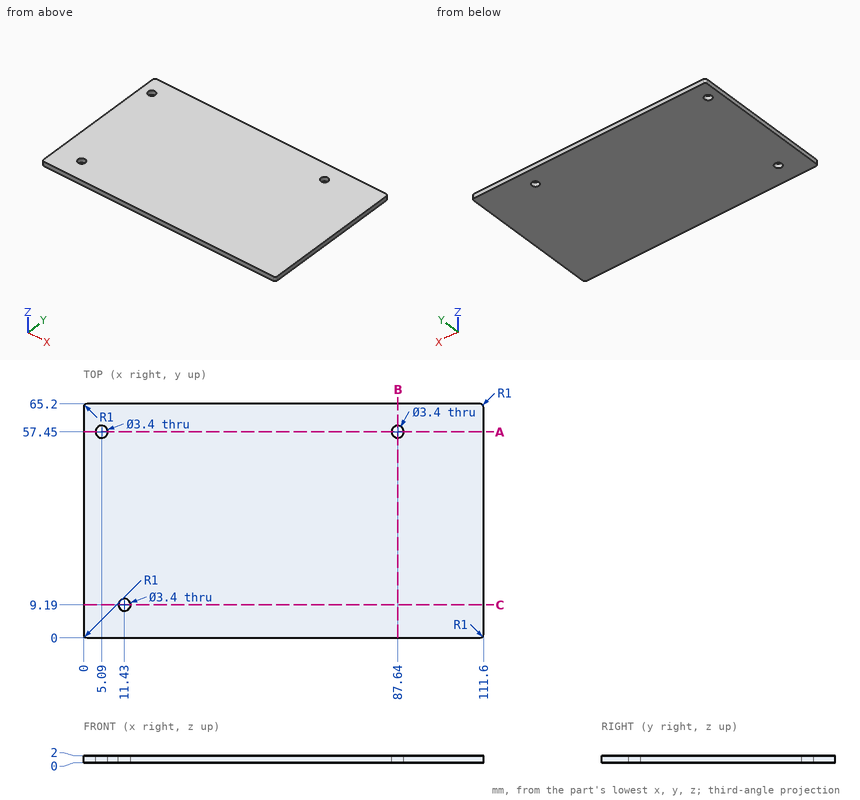
Answer from the drawing. Dimensions are ordinates in mm from the lowest x, y and z of the part. Coordinates: 2 decimals unless noted, no trailing zeros. Write each loop counter-clockwise with the first axis right and the second up, starting at its lowest first coordinate (ties: lowest second). Pieces come first, ordered by that corner, then holes. Notation, with made-up numbers: M 56.5,74.5 L 101.5,74.5 A21 ccw 101.5,94.5 Z; hole C -13.75,-39 d11. An arc over 180 degrees is marked long. Put each result on its own line as item: value. Start each with the question number.
1. Consider line 1 (X direction, y = 57.45, z = 0.6); line 2 (Y direction, x = 87.64, z = 0.8); line 3 (Y direction, x = 11.43, z = 0.8). Determine where each line is inside the solid, lowest interval first. Write a range as from..to.
2. A cutting plane is placed at C-C on y = 9.19. Write down the section's boundary in (x, z).
3. A cutting plane is placed at A-A on y = 57.45. Write down the section's boundary in (x, z), then the cut area to 3 significant figures.
4. A cutting plane is placed at B-B on x = 87.64. Write down the section's boundary in (y, z).
Resolved:
1. line 1: x = 0..3.39, 6.79..85.94, 89.34..111.6
1. line 2: y = 0..55.75, 59.15..65.2
1. line 3: y = 0..7.49, 10.89..65.2
2. outline: M 0,0 L 9.73,0 L 9.73,2 L 0,2 Z; M 13.13,0 L 111.6,0 L 111.6,2 L 13.13,2 Z
3. outline: M 0,0 L 3.39,0 L 3.39,2 L 0,2 Z; M 6.79,0 L 85.94,0 L 85.94,2 L 6.79,2 Z; M 89.34,0 L 111.6,0 L 111.6,2 L 89.34,2 Z
3. area: 210 mm2
4. outline: M 0,0 L 55.75,0 L 55.75,2 L 0,2 Z; M 59.15,0 L 65.2,0 L 65.2,2 L 59.15,2 Z
